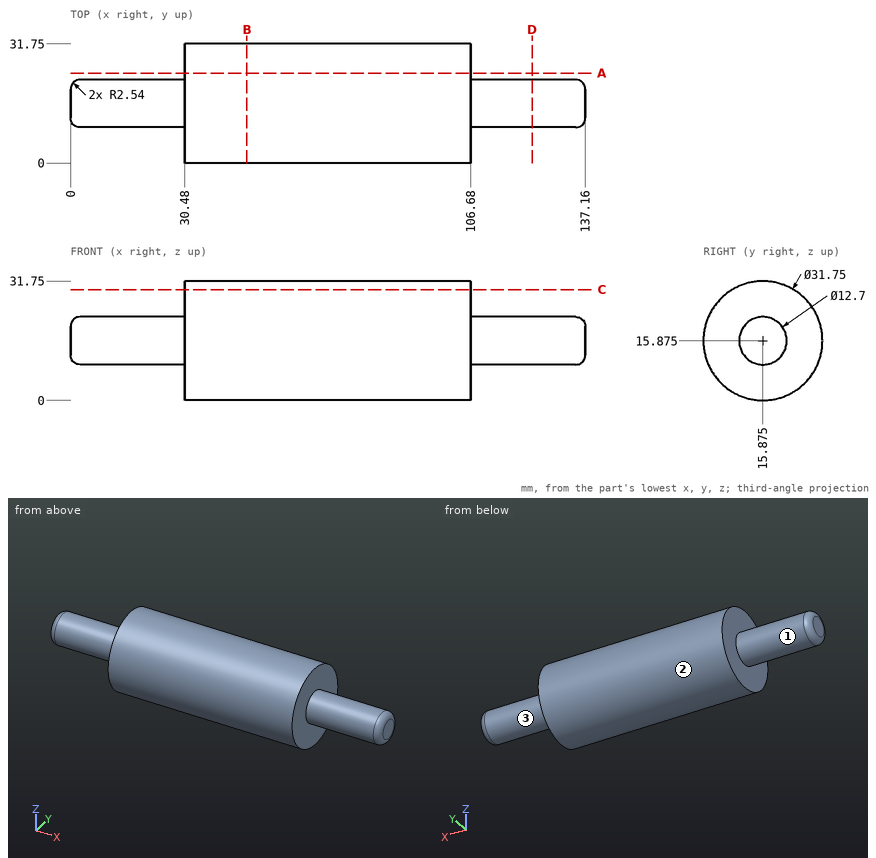
Check sheet for the drawn part. Datum: minimum x, y, z corner. Units: mm. A direction names the side the tool comes from. Coordinates: 2 decimals unless noted, no trailing zeros. Write each loop counter-clockwise with the first axis right and the second up, starting at its lowest first coordinate (ties: lowest second). Pieces come first, ordered by that corner, then holes. Notation, with made-up numbers: (47.5, 62.25) - (84.5, 62.25) arc R25 ccw to (84.5, 75.25) - close; hole circle Ø2 at (8, -12.5). An arc over 180 degrees is marked (long way). Answer as a JSON object with one key per item and string values.
(1) Gauge pin test, flat ends, axial feed: pin 1 Ø3 at (y, z) = (16, 22.5) entering from +X; pin 2 Ø9.5 at (y, z) = (19, 22) entering from -X; pin 3 Ø3 at (x, z) = (83.5, 28.5) entering from -Y; pin 4 Ø4 at (y, z) = (15, 5) entering from +X. Record the tip position at first contact, or that the pin passes through.
Report:
{"pin 1": "x = 136.79", "pin 2": "x = 0", "pin 3": "y = 4.55", "pin 4": "x = 106.68"}
(2) Tool access check on the marked faces 1, 2 and 3. Record the directions out of +Z, -Z, +X, -X, +Y, -Y that give a thin tool (end or side, any length) a straight path to the whole face; none if there is none.
Report:
{"face 1": "-X", "face 2": "+X, -X", "face 3": "+X"}
(3) Thickness scan on line 1 along X through (y, z) = (10, 13); line 2 along Y through (x, z) = (80, 15); line 3 along Z through (x, y) = (65.5, 25). Record the ranges inside material, lowest first.
Report:
{"line 1": "30.48 to 106.68", "line 2": "0.02 to 31.73", "line 3": "2.88 to 28.87"}
(4) Cross-section at B-B on x = 47. Record the cut outline in (y, z) (3 decimals), plus the area to 3 significant figures.
Report:
{"outline": "circle Ø31.75 at (15.875, 15.875)", "area": "792 mm^2"}
(5) Cross-section at A-A on y = 24. Record the cut outline in (x, z).
Report:
{"outline": "(30.48, 2.24) - (106.68, 2.24) - (106.68, 29.51) - (30.48, 29.51) - close"}
(6) Cross-section at C-C on z = 29.5. Record the cut outline in (x, y), plus the area to 3 significant figures.
Report:
{"outline": "(30.48, 7.73) - (106.68, 7.73) - (106.68, 24.02) - (30.48, 24.02) - close", "area": "1,240 mm^2"}
(7) Cross-section at D-D on x = 123. Record the cut outline in (y, z) (3 decimals).
Report:
{"outline": "circle Ø12.7 at (15.875, 15.875)"}
